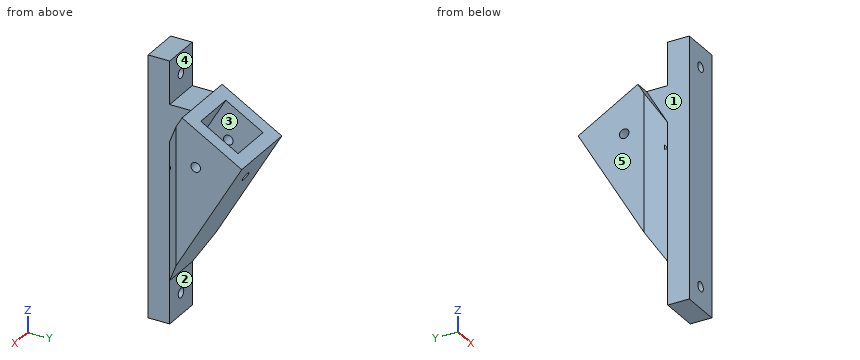
Autodesk Inventor part; units mm, degrees
ref_plane "YZ Plane" through (0, 0, 0) normal (1, 0, 0) x (0, 1, 0)
ref_plane "XZ Plane" through (0, 0, 0) normal (0, 1, 0) x (-1, 0, 0)
ref_plane "XY Plane" through (0, 0, 0) normal (0, 0, 1) x (1, 0, 0)
sketch "Sketch1" plane through (0, 0, 0) normal (1, 0, 0) x (0, 1, 0)
  line L0 (0, 0) -> (12.4509, 21.5656)
  line L1 (12.4509, 21.5656) -> (47.6462, 1.2456)
  line L2 (0, -101.8491) -> (0, 42.1347)
  line L3 (47.6462, 1.2456) -> (0, -81.28)
  line L4 (0, 0) -> (0, -81.28)
  line L5 (19.05, 17.7556) -> (0, -15.24) construction
  dimension "d0" = 40.64
  dimension "d1" = 30
  dimension "d5" = 7.62
  dimension "d6" = 38.1
extrude "Extrusion1" add sketch "Sketch1" along normal mid plane 40.64
sketch "Sketch2" plane through (-20.32, 12.4509, 21.5656) normal (0, 0.5, 0.8660254) x (1, 0, 0)
  line L0 (0, 0) -> (40.64, 0) construction
  line L1 (40.64, 0) -> (40.64, 40.64) construction
  line L2 (0, 0) -> (40.64, 40.64) construction
  line L3 (40.64, 40.64) -> (0, 40.64) construction
  line L4 (0, 40.64) -> (40.64, 0) construction
  line L5 (7.62, 7.62) -> (33.02, 7.62)
  line L6 (33.02, 7.62) -> (33.02, 33.02)
  line L7 (33.02, 33.02) -> (7.62, 33.02)
  line L8 (7.62, 33.02) -> (7.62, 7.62)
  line L9 (7.62, 7.62) -> (33.02, 33.02) construction
  line L10 (33.02, 7.62) -> (7.62, 33.02) construction
  point P0 (20.32, 0)
  point P1 (20.32, 20.32)
  dimension "d7" = 25.4
extrude "Extrusion2" cut sketch "Sketch2" against normal blind 38.1
sketch "Sketch3" plane through (0, 0, 0) normal (1, 0, 0) x (0, 1, 0)
  line L0 (12.4509, 21.5656) -> (0, 0)
  line L1 (0, 0) -> (0, -81.28)
  line L2 (0, -81.28) -> (47.6462, 1.2456)
  line L3 (21.997, -27.94) -> (0, -15.24)
  line L4 (19.05, 17.7556) -> (0, -15.24)
  line L5 (0, 0) -> (0, -81.28)
  line L6 (12.4509, 21.5656) -> (-1.0999, 21.5656) construction
  line L7 (0, 0) -> (12.4509, 21.5656)
  line L8 (0, 0) -> (0, 46.9656)
  line L9 (47.6462, 1.2456) -> (0, -81.28)
  line L10 (0, -81.28) -> (0, -106.68)
  line L11 (0, -137.7901) -> (0, 79.9807)
  line L12 (0, 46.9656) -> (-12.7, 46.9656)
  line L13 (-12.7, 46.9656) -> (-12.7, -106.68)
  line L14 (-12.7, -106.68) -> (0, -106.68)
  point P0 (1.0999, -13.335)
  dimension "d10" = 25.4
  dimension "d11" = 25.4
  dimension "d12" = 12.7
  dimension "supportBaseLength" = 153.6456
extrude "Extrusion3" add sketch "Sketch3" along normal mid plane 22.86
sketch "Sketch5" plane through (0, 0, 0) normal (1, 0, 0) x (0, 1, 0)
  line L0 (0, 0) -> (12.4509, 21.5656)
  line L1 (0, 46.9656) -> (0, 0)
  line L2 (12.4509, 21.5656) -> (47.6462, 1.2456)
  line L3 (12.4509, 21.5656) -> (0, 21.5656)
  line L4 (0, 0) -> (12.4509, 21.5656)
extrude "Extrusion5" add sketch "Sketch5" along normal mid plane 22.86
sketch "Sketch4" plane through (0, 0, 0) normal (0, 0, 1) x (1, 0, 0)
  line L0 (20.32, 47.6462) -> (-20.32, 47.6462)
  line L1 (20.32, 0) -> (20.32, 47.6462)
  line L2 (20.32, 0) -> (11.43, 0)
  line L3 (11.43, 0) -> (-11.43, 0)
  line L4 (-11.43, 0) -> (-20.32, 0)
  line L5 (-20.32, 47.6462) -> (-20.32, 0)
  line L6 (-11.43, 0) -> (-11.43, -12.7)
  line L7 (11.43, -12.7) -> (-11.43, -12.7)
  line L8 (11.43, -12.7) -> (11.43, 0)
  line L9 (-11.43, 0) -> (-20.32, 8.89)
  line L10 (-20.32, 47.6462) -> (-20.32, 0)
  line L11 (-20.32, 8.89) -> (-20.32, 0)
  line L12 (0, 0) -> (0, 47.6462) construction
  line L13 (11.43, 0) -> (20.32, 0)
  line L14 (11.43, 0) -> (20.32, 8.89)
  line L15 (20.32, 8.89) -> (20.32, 0)
  dimension "d15" = 45
extrude "Extrusion4" cut sketch "Sketch4" against normal up to surface (153.6456 mm away) from surface at 46.9656 contours L1 L2 L14 | L9 L4 L5
sketch "Sketch6" plane through (-11.43, 0, 46.9656) normal (0, 1, 0) x (1, 0, 0)
  line L0 (22.86, 153.6456) -> (0, 153.6456) construction
  line L1 (11.43, 153.6456) -> (11.43, 0) construction
  line L2 (22.86, 0) -> (0, 0) construction
  point P0 (11.43, 46.9656)
  point P1 (11.43, 140.9456)
  point P2 (11.43, 12.7)
  dimension "d21" = 12.7
  dimension "d22" = 12.7
hole "Hole1" at (0, 0, -93.98) at (0, 0, 34.2656) direction (0, -1, 0) diameter 5.6134 end through all
sketch "Sketch9" plane through (0, 0, 0) normal (1, 0, 0) x (0, 1, 0)
  line L0 (1.27, -13.0403) -> (1.27, -15.9732)
  line L1 (1.27, -15.9732) -> (21.997, -27.94)
  line L2 (41.047, 5.0556) -> (21.997, -27.94)
  line L3 (19.05, 17.7556) -> (41.047, 5.0556)
  line L4 (19.05, 17.7556) -> (1.27, -13.0403)
  line L5 (30.0485, 11.4056) -> (10.9985, -21.59) construction
  line L6 (1.27, -15.9732) -> (21.997, -27.94) construction
  circle A0 centre (20.5235, -5.0922) radius 2.8067
  point P0 (0, 0)
  dimension "d30" = 5.6134
extrude "Extrusion6" cut sketch "Sketch9" along normal through all both and the other way through all contours A0
sketch "Sketch10" plane through (-20.32, 47.6462, 1.2456) normal (0, 0.8660254, -0.5) x (1, 0, 0)
  line L0 (7.62, 0) -> (33.02, 0) construction
  line L1 (20.32, 0) -> (20.32, 77.7875) construction
  point P0 (20.32, 24.9018)
  point P1 (20.32, 19.05)
  dimension "d33" = 19.05
hole "Hole2" at (0, 38.1212, -15.2522) direction (0, -0.8660254, 0.5) diameter 5.6134 depth 7.62
equation "\"d0\" = widthToSupportExtrusion"
equation "\"d1\" = attachementAngle"
equation "\"d6\" = insertDepth"
equation "\"d2\" = widthToSupportExtrusion"
equation "\"d7\" = extrusionSize"
equation "\"d8\" = insertDepth"
equation "\"d12\" = supportBaseDepth"
equation "\"d13\" = supportBaseWidth"
equation "\"attachementAngle\" = 30deg"
equation "\"extrusionSize\" = 25.4"
equation "\"wallThickness\" = 6.35"
equation "\"slipClearance\" = 1.27"
equation "\"insertForExtrusion\" = extrusionSize + 2 * slipClearance"
equation "\"widthToSupportExtrusion\" = insertForExtrusion + 2 * wallThickness"
equation "\"insertDepth\" = 38.1"
equation "\"supportBaseWidth\" = 22.86"
equation "\"supportBaseDepth\" = 12.7"
properties part number "30DegreeAttachementV02"
Part model, mm, in its own coordinate system. Face numbers are marked on the shaded views. A direction names the side the tool comes from. Coordinates: 2 decimals unless noted, no trailing zeros. Write each loop counter-clockwise with the first axis right and the second up, starting at its lowest first coordinate (ties: lowest second). Pieces come first, ordered by that corner, then holes. Notation, with made-up numbers: M -25,41.5 L 24,41.5 A22 ccw 24,56.5 Z; hole C 17.25,12.25 d9. An arc over 180 degrees is marked long. Return JSON: item names as keys, results as strings.
1. Saw through at A-A, the plane z = -93.98. Write the cut outline in (x, y), then the cut area to 3 significant figures.
Determined:
{"outline": "M -11.43,-12.7 L -2.81,-12.7 L -2.81,0 L -11.43,0 Z; M 2.81,-12.7 L 11.43,-12.7 L 11.43,0 L 2.81,0 Z", "area": "219 mm²"}
2. Probe L1, parallel to Z at x = 0, y = -8; L2, parallel to X at y = -2.5, z = 34; L3, parallel to Y at x = -0.5, z = -22. List the from-to ranges inside material, lowest first.
Determined:
{"L1": "-106.68 to -96.79, -91.17 to 31.46, 37.07 to 46.97", "L2": "-11.43 to -2.79, 2.79 to 11.43", "L3": "-12.7 to 11.7, 25.43 to 34.23"}
3. Saw through at C-C, the plane y = 28. Write the cut outline in (x, z), then the cut area to 3 significant figures.
Determined:
{"outline": "M -20.32,-32.78 L 20.32,-32.78 L 20.32,12.59 L 12.7,12.59 L 12.7,-17.54 L -12.7,-17.54 L -12.7,12.59 L -20.32,12.59 Z", "area": "1,080 mm²"}
4. Pull direction X, two halves, no side cores. Call the marked faces 1, 2 and 3: pulls with the +X half, pulls with the -X half, needs draft (parallel to the pull), parting line crosses it, or undercut.
Determined:
{"face 1": "pulls with the -X half", "face 2": "needs draft", "face 3": "undercut"}
5. Saw through at B-B, the plane x = 0. Count the separate pieces of the cut face and the enclosed holes in it, then the cut area to 3 significant figures.
Determined:
{"separate pieces": "4", "enclosed holes": "0", "area": "3,370 mm²"}
6. Saw through at D-D, the plane z = -42.5. Write the cut outline in (x, y), then the cut area to 3 significant figures.
Determined:
{"outline": "M -20.32,8.89 L -11.43,0 L -11.43,-12.7 L 11.43,-12.7 L 11.43,0 L 20.32,8.89 L 20.32,22.39 L -20.32,22.39 Z", "area": "1,120 mm²"}
7. 3-axis set-ups, long thin cutter, end or side, ignore diameter. For the marked faces 4 and 5: which of +Z, -Z, +X, -X, +Y, -Y reach the whole face in a straight line?
Determined:
{"face 4": "+Z, +X, -X, +Y", "face 5": "+Z, -Z, -X, +Y, -Y"}
8. Flat gauge pins, fed straight in: pin 1 Ø2 at (x, z) = (12, 21.5) entering from -Y; pin 2 Ø8 at (y, z) = (-3.5, -14.5) entering from -X; pin 3 Ø1 at (x, y) = (10, 32.5) entering from +Z; pin 4 Ø1.5 at (x, y) = (-6.5, 28) entering from +Z. Where does each tip first touch, or does it go through?
Determined:
{"pin 1": "y = -12.7", "pin 2": "x = -11.93", "pin 3": "z = -8.88", "pin 4": "z = -16.24"}
